```python
from build123d import *

# Parameters (mm, degrees)
BASE_FLANGE1_DEPTH     = 1.5
EDGE_FLANGE1_DEPTH     = 175
EDGE_FLANGE1_2_DEPTH   = 175
EDGE_FLANGE2_OUTLINE_W = 1.5
EDGE_FLANGE2_OUTLINE_H = 25
EDGE_FLANGE2_DEPTH     = 50
EDGE_FLANGE2_2_DEPTH   = 175
EDGE_FLANGE2_3_DEPTH   = 175
EDGE_FLANGE2_START     = 68
EDGE_FLANGE2_4_DEPTH   = 4
EDGE_FLANGE3_DEPTH     = 122
SKETCH15_R             = 2.2
CUT_EXTRUDE1_DEPTH     = 10
FILLET1_R              = 5
CUT_EXTRUDE2_DEPTH     = 10
CUT_EXTRUDE3_DEPTH     = 10
SKETCH18_R             = 4
CUT_EXTRUDE4_DEPTH     = 10


with BuildPart() as part:
    # Base-Flange1: sheet metal written as solids
    # Sketch1 → Base-Flange1 (new body)
    with BuildSketch(Plane.XY):
        with BuildLine():
            Line((0, 0), (0, 47.9))
            Line((0, 47.9), (175, 47.9))
            Line((175, 47.9), (175, 27.9))
            Line((175, 27.9), (67, 27.9))
            ThreePointArc((67, 27.9), (56.393398282, 23.506601718), (52, 12.9))
            Line((52, 12.9), (52, 0))
            Line((52, 0), (0, 0))
        make_face()
    extrude(amount=-BASE_FLANGE1_DEPTH)

    # Edge-Flange1: read off the stored shape, not the designer's step
    # Edge-Flange1 outline → Edge-Flange1 (cut)
    with BuildSketch(Plane.YZ):
        with BuildLine():
            ThreePointArc((45.0745166, 0), (46.299103584, -0.243585496), (47.3372583, -0.9372583))
            Line((47.3372583, -0.9372583), (47.9, -1.5))
            Line((47.9, -1.5), (47.9, 0))
            Line((47.9, 0), (45.0745166, 0))
        make_face()
    extrude(amount=EDGE_FLANGE1_DEPTH, mode=Mode.SUBTRACT)

    # Edge-Flange1 2 outline → Edge-Flange1 2 (add)
    with BuildSketch(Plane.YZ):
        with BuildLine():
            Line((71.839339828, -25.439339828), (47.9, -1.5))
            Line((47.9, -1.5), (45.0745166, -1.5))
            ThreePointArc((45.0745166, -1.5), (45.725078435, -1.629404795), (46.276598128, -1.997918472))
            Line((46.276598128, -1.997918472), (70.778679656, -26.5))
            Line((70.778679656, -26.5), (71.839339828, -25.439339828))
        make_face()
    extrude(amount=EDGE_FLANGE1_2_DEPTH)

    # Edge-Flange2 2 outline → Edge-Flange2 2 (cut)
    with BuildSketch(Plane.YZ):
        with BuildLine():
            ThreePointArc((69.841421356, -23.441421356), (70.53509416, -24.479576072), (70.778679656, -25.704163056))
            Line((70.778679656, -25.704163056), (70.778679656, -26.5))
            Line((70.778679656, -26.5), (71.839339828, -25.439339828))
            Line((71.839339828, -25.439339828), (69.841421356, -23.441421356))
        make_face()
    extrude(amount=EDGE_FLANGE2_2_DEPTH, mode=Mode.SUBTRACT)



with BuildPart() as body_2:
    # Edge-Flange2: read off the stored shape, not the designer's step
    # Edge-Flange2 outline → Edge-Flange2 (new body)
    with BuildSketch(Plane.YZ):
        with Locations((70.028679656, -57.5)):
            Rectangle(EDGE_FLANGE2_OUTLINE_W, EDGE_FLANGE2_OUTLINE_H)
    extrude(amount=EDGE_FLANGE2_DEPTH)


with BuildPart() as part_1:
    add(part.part)

    add(body_2.part)  # Edge-Flange2 3 merges body 2
    # Edge-Flange2 3 outline → Edge-Flange2 3 (add)
    with BuildSketch(Plane.YZ):
        with BuildLine():
            Line((70.778679656, -45), (70.778679656, -26.5))
            Line((70.778679656, -26.5), (68.780761184, -24.502081528))
            ThreePointArc((68.780761184, -24.502081528), (69.149274862, -25.053601221), (69.278679656, -25.704163056))
            Line((69.278679656, -25.704163056), (69.278679656, -45))
            Line((69.278679656, -45), (70.778679656, -45))
        make_face()
    extrude(amount=EDGE_FLANGE2_3_DEPTH)

    # Edge-Flange2 4 outline → Edge-Flange2 4 (cut)
    with BuildSketch(Plane(origin=(0, 0, 0), x_dir=(1, 0, 0), z_dir=(0, 1, 0)).offset(EDGE_FLANGE2_START)):
        with BuildLine():
            ThreePointArc((50, 45), (51.5, 43.5), (53, 45))
            Line((53, 45), (50, 45))
        make_face()
    extrude(amount=EDGE_FLANGE2_4_DEPTH, mode=Mode.SUBTRACT)

    # Edge-Flange3: sheet metal written as solids
    # Edge-Flange3 section (on a plane across the edge) → Edge-Flange3 (add)
    with BuildSketch(Plane(origin=(53, 69.278679656, -46.7), x_dir=(0, 0, 1), z_dir=(1, 0, 0))):
        with BuildLine():
            Line((-1.5, 1.7), (-1.5, 6.5))
            Line((-1.5, 6.5), (0, 6.5))
            Line((0, 6.5), (0, 1.7))
            ThreePointArc((0, 1.7), (0.497918472, 0.497918472), (1.7, 0))
            Line((1.7, 0), (1.7, -1.5))
            ThreePointArc((1.7, -1.5), (-0.5627417, -0.5627417), (-1.5, 1.7))
        make_face()
    extrude(amount=EDGE_FLANGE3_DEPTH)

    # Sketch15 → Cut-Extrude1 (cut)
    with BuildSketch(Plane(origin=(0, 70.778679656, 0), x_dir=(1, 0, 0), z_dir=(0, 1, 0))):
        with Locations(Location((25, 45, 0), (0, 0, 270))):
            Circle(SKETCH15_R)
        with Locations(Location((25, 60, 0), (0, 0, 270))):
            Circle(SKETCH15_R)
    extrude(amount=-CUT_EXTRUDE1_DEPTH, mode=Mode.SUBTRACT)

    # Fillet1
    fillet1_edges = [part_1.edges().sort_by_distance(p)[0] for p in [
        (52, 0, -0.75),
        (0, 0, -0.75),
        (50, 70.028679656, -70),
        (0, 70.028679656, -70),
        (53, 62.778679656, -47.45),
    ]]
    fillet(fillet1_edges, radius=FILLET1_R)

    # Sketch16 → Cut-Extrude2 (cut)
    with BuildSketch(Plane.XY):
        with BuildLine():
            Line((28.75, 30), (28.75, 28))
            ThreePointArc((28.75, 28), (26, 25.25), (23.25, 28))
            Line((23.25, 28), (23.25, 30))
            ThreePointArc((23.25, 30), (26, 32.75), (28.75, 30))
        make_face()
        with BuildLine():
            Line((28.75, 15), (28.75, 13))
            ThreePointArc((28.75, 13), (26, 10.25), (23.25, 13))
            Line((23.25, 13), (23.25, 15))
            ThreePointArc((23.25, 15), (26, 17.75), (28.75, 15))
        make_face()
    extrude(amount=-CUT_EXTRUDE2_DEPTH, mode=Mode.SUBTRACT)

    # Sketch17 → Cut-Extrude3 (cut)
    with BuildSketch(Plane(origin=(0, 23.2, 23.2), x_dir=(1, 0, 0), z_dir=(0, 0.7071067811865438, 0.7071067811865513))):
        with BuildLine():
            Line((150.833333333, 57.548084348), (199.166666667, 57.548084348))
            ThreePointArc((199.166666667, 57.548084348), (206.666666667, 50.048084348), (199.166666667, 42.548084348))
            Line((199.166666667, 42.548084348), (150.833333333, 42.548084348))
            ThreePointArc((150.833333333, 42.548084348), (143.333333333, 50.048084348), (150.833333333, 57.548084348))
        make_face()
        with BuildLine():
            Line((67.5, 57.548084348), (115.833333333, 57.548084348))
            ThreePointArc((115.833333333, 57.548084348), (123.333333333, 50.048084348), (115.833333333, 42.548084348))
            Line((115.833333333, 42.548084348), (67.5, 42.548084348))
            ThreePointArc((67.5, 42.548084348), (60, 50.048084348), (67.5, 57.548084348))
        make_face()
    extrude(amount=-CUT_EXTRUDE3_DEPTH, mode=Mode.SUBTRACT)

    # Sketch18 → Cut-Extrude4 (cut)
    with BuildSketch(Plane(origin=(0, 23.2, 23.2), x_dir=(1, 0, 0), z_dir=(0, 0.7071067811865438, 0.7071067811865513))):
        with Locations(Location((13.5, 50.048084348, 0), (0, 0, 270))):
            Circle(SKETCH18_R)
        with Locations(Location((36.5, 50.048084348, 0), (0, 0, 270))):
            Circle(SKETCH18_R)
        with Locations(Location((25, 50.048084348, 0), (0, 0, 270))):
            Circle(SKETCH18_R)
    extrude(amount=-CUT_EXTRUDE4_DEPTH, mode=Mode.SUBTRACT)

    # Mirror1: part across plane


with BuildPart() as part_2:
    add(part_1.part)
    add(part_1.part.mirror(Plane(origin=(175, 71.839339828, -25.439339828), x_dir=(0, 0, 1), z_dir=(-1, 0, 0))))


solid = part_2.part
```
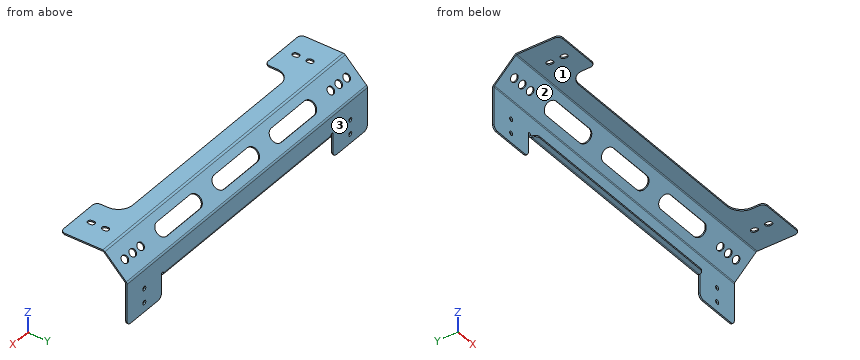
The listing builds one solid part. Answer for the finished solid, in the listing's coordinates (mm). Face numbers are marked on the shaded views. A direction names the side the tool comes from. Give positions to 0.01 mm unless a question says otherwise; leave off trailing zeros. Order: outer loops, then holes, each group sorted by start corner. A loop starts at its lowest first (then second) coordinate and runs counter-clockwise, first axis right, second up. Notation, with made-up numbers: (30, -12.75) - (64, -12.75) arc R25 ccw to (64, 14.25) - close; hole circle Ø6 at (36, 13.5). An arc over 180 degrees is marked (long way). Use one line per item in the form item = value. Start each with the question number.
(1) A cutting plane is placed at C-C, the plane y = 38.5. Write down the section's boundary in (x, z).
(2) Consider line 1 (X direction, y = 70.55, z = -45); line 2 (X direction, y = 70.45, z = -60); line 3 (Z direction, x = 325, y = 70.45). Determine where each line is inside the solid, lowest interval first. Write a range as from..to.
(3) A cutting plane is placed at B-B, the plane x = 220.5. Write down the section's boundary in (y, z), then the cut area to 3 significant figures.
(4) A cutting plane is placed at A-A, the plane x = 275.5. Write down the section's boundary in (y, z), then the cut area to 3 significant figures.
(5) For the marked faces 1, 2 and 3, determine the directions among +Z, -Z, +X, -X, +Y, -Y from which every point of the face is accessible in a straight line to the end or side of a thin tool.
(6) Flat-ended cylindrical pins translate along their axes: pin 1 Ø2.5 at (x, z) = (25, -60) entering from +Y; pin 2 Ø8 at (x, y) = (300, 55) entering from +Z; pin 3 Ø6 at (x, y) = (157, 60) entering from -Z; pin 4 Ø5 at (x, z) = (325, -60) entering from -Y. Find the tip coordinate at first contact, or state that the pin passes through.
Ans:
q1.outline = (0, -1.5) - (350, -1.5) - (350, 0) - (0, 0) - close
q2.line_1 = 0..22.8, 27.2..50, 53..297, 300..322.8, 327.2..350
q2.line_2 = 0..22.8, 27.2..50, 300..322.8, 327.2..350
q2.line_3 = -70..-62.2, -57.8..-47.2, -42.8..-24.29
q3.outline = (27.9, -1.5) - (45.07, -1.5) arc R1.7 cw to (46.28, -2) - (68.78, -24.5) arc R1.7 cw to (69.28, -25.7) - (69.28, -45) arc R1.7 cw to (67.58, -46.7) - (62.78, -46.7) - (62.78, -48.2) - (67.58, -48.2) arc R3.2 ccw to (70.78, -45) - (70.78, -25.7) arc R3.2 ccw to (69.84, -23.44) - (47.34, -0.94) arc R3.2 ccw to (45.07, 0) - (27.9, 0) - close
q3.area = 121 mm^2
q4.outline = (27.9, -1.5) - (45.07, -1.5) arc R1.7 cw to (46.28, -2) - (52.23, -7.95) - (53.29, -6.89) - (47.34, -0.94) arc R3.2 ccw to (45.07, 0) - (27.9, 0) - close; (62.78, -48.2) - (67.58, -48.2) arc R3.2 ccw to (70.78, -45) - (70.78, -25.7) arc R3.2 ccw to (69.84, -23.44) - (63.89, -17.49) - (62.83, -18.55) - (68.78, -24.5) arc R1.7 cw to (69.28, -25.7) - (69.28, -45) arc R1.7 cw to (67.58, -46.7) - (62.78, -46.7) - close
q4.area = 98.7 mm^2
q5.face_1 = -Z, +X, -X, -Y
q5.face_2 = +X, -X, -Y
q5.face_3 = +Z, -Z, +X, -X, +Y
q6.pin_1 = through
q6.pin_2 = -4.6
q6.pin_3 = -48.2
q6.pin_4 = 69.28
